Here's how the part is built. I have some questions about the finished solid (model axes, mm). A direction names the side the tool comes from. Coordinates: 2 decimals unless noted, no trailing zeros. Write each loop counter-clockwise with the first axis right and the second up, starting at its lowest first coordinate (ties: lowest second). Pieces come first, ordered by that corner, then holes.
```python
from build123d import *

# Parameters (mm, degrees)
BOSS_EXTRUDE1_DEPTH = 8
CIRPATTERN1_COUNT   = 4


# Read off the part's stored shape, not the designer's step: CSK for M3 Hex Socket Countersunk Cap Screw1
with BuildPart() as part:
    # Sketch2 → Boss-Extrude1 (new body)
    with BuildSketch(Plane(origin=(0, 0, 0), x_dir=(1, 0, 0), z_dir=(0, 1, 0))):
        with BuildLine():
            Line((6, -29.393876913), (102, -9.797958971))
            ThreePointArc((102, -9.797958971), (110, 0), (102, 9.797958971))
            Line((102, 9.797958971), (6, 29.393876913))
            ThreePointArc((6, 29.393876913), (-30, 0), (6, -29.393876913))
        make_face()
        with BuildLine():
            Line((37.941125497, -12.667714712), (100, 0))
            Line((100, 0), (37.941125497, 12.667714712))
            ThreePointArc((37.941125497, 12.667714712), (40, 0), (37.941125497, -12.667714712))
        make_face(mode=Mode.SUBTRACT)
    boss_extrude1 = extrude(amount=BOSS_EXTRUDE1_DEPTH)

    # CirPattern1: Boss-Extrude1 ×4 about axis
    cirpattern1_axis = Axis((0, 0, 0), (0, 1, 0))
    for i in range(1, CIRPATTERN1_COUNT):
        add(boss_extrude1.rotate(cirpattern1_axis, i * 360 / CIRPATTERN1_COUNT))

    # CSK for M3 Hex Socket Countersunk Ca 2 → CSK for M3 Hex Socket Countersunk Cap Screw1 (revolve, cut)
    with BuildSketch(Plane(origin=(-11.258330249, 0, -6.5), x_dir=(1, 0, 0), z_dir=(0, 0, 1))):
        Polygon((1.8, 1.56), (1.8, 8), (0, 8), (0, 0), (3.36, 0), align=None)
    revolve(axis=Axis((-11.258330249, 0, -6.5), (0, 1, 0)), mode=Mode.SUBTRACT)

    # CSK for M3 Hex Socket Countersunk Ca 3 o → CSK for M3 Hex Socket Countersunk Ca 3 (revolve, cut)
    with BuildSketch(Plane(origin=(-11.258330249, 0, 6.5), x_dir=(1, 0, 0), z_dir=(0, 0, 1))):
        Polygon((1.8, 1.56), (1.8, 8), (0, 8), (0, 0), (3.36, 0), align=None)
    revolve(axis=Axis((-11.258330249, 0, 6.5), (0, 1, 0)), mode=Mode.SUBTRACT)

    # CSK for M3 Hex Socket Countersunk Ca 4 o → CSK for M3 Hex Socket Countersunk Ca 4 (revolve, cut)
    with BuildSketch(Plane.XY.offset(13)):
        Polygon((1.8, 1.56), (1.8, 8), (0, 8), (0, 0), (3.36, 0), align=None)
    revolve(axis=Axis((0, 0, 13), (0, 1, 0)), mode=Mode.SUBTRACT)

    # CSK for M3 Hex Socket Countersunk Ca 5 o → CSK for M3 Hex Socket Countersunk Ca 5 (revolve, cut)
    with BuildSketch(Plane(origin=(11.258330249, 0, 6.5), x_dir=(1, 0, 0), z_dir=(0, 0, 1))):
        Polygon((1.8, 1.56), (1.8, 8), (0, 8), (0, 0), (3.36, 0), align=None)
    revolve(axis=Axis((11.258330249, 0, 6.5), (0, 1, 0)), mode=Mode.SUBTRACT)

    # CSK for M3 Hex Socket Countersunk Ca 6 o → CSK for M3 Hex Socket Countersunk Ca 6 (revolve, cut)
    with BuildSketch(Plane(origin=(11.258330249, 0, -6.5), x_dir=(1, 0, 0), z_dir=(0, 0, 1))):
        Polygon((1.8, 1.56), (1.8, 8), (0, 8), (0, 0), (3.36, 0), align=None)
    revolve(axis=Axis((11.258330249, 0, -6.5), (0, 1, 0)), mode=Mode.SUBTRACT)

    # CSK for M3 Hex Socket Countersunk Ca 7 o → CSK for M3 Hex Socket Countersunk Ca 7 (revolve, cut)
    with BuildSketch(Plane.XY.offset(-13)):
        Polygon((1.8, 1.56), (1.8, 8), (0, 8), (0, 0), (3.36, 0), align=None)
    revolve(axis=Axis((0, 0, -13), (0, 1, 0)), mode=Mode.SUBTRACT)


solid = part.part
```
1) Imagine slicing it at D-D on z = 29. Please give me the cut outline in (x, y), then the cut area to 3 significant figures.
Values follow:
outline: (-24.7, 0) - (24.7, 0) - (24.7, 8) - (-24.7, 8) - close
area: 395 mm2
2) Will these pins go through, and if not, where does the flat tip stop? pin 1 (4 mm diameter, centred on y = 2.5, z = -60, fed in from -X); pin 2 (1 mm diameter, centred on x = -7, y = 5, fed in from +Z); pin 3 (6 mm diameter, centred on x = -11.26, z = -6.5, fed in from +Y).
Values follow:
pin 1: stops at x = -18.78
pin 2: stops at z = 107.6
pin 3: stops at y = 8
3) On a 3-axis mill with a long thin cutter (end or side, diameter ignored), from which of +Z, -Z, +X, -X, +Y, -Y can I reach the whole of each face in a straight line? I mean faces 5 (the face through (69.405, 3.944, -6.245)), 6 (the face through (17.722, 3.944, -63.178)). Say none if no direction works.
Values follow:
face 5: +Y, -Y
face 6: -Z, +X, +Y, -Y
4) Imagine slicing it at A-A on x = 96. Please give me the cut outline in (y, z).
Values follow:
outline: (0, -11.02) - (8, -11.02) - (8, -0.82) - (0, -0.82) - close; (0, 0.82) - (8, 0.82) - (8, 11.02) - (0, 11.02) - close
5) We'd pull the mould along X, two halves only. Please class faces 1 (the face through (-68.54, 3.94, -6.42)), 2 (the face through (-17.504, 3.944, -64.25)), 3 (the face through (0, 4, -110)), 4 (the face through (68.54, 3.94, 6.42)): pulls with the +X half, pulls with the -X half, needs draft (parallel to the pull), parting line crosses it, or undercut.
Values follow:
face 1: undercut
face 2: pulls with the -X half
face 3: parting line crosses it
face 4: undercut
6) Imagine slicing it at B-B on y = 5. Count the separate pieces of the cut face and the enclosed holes in it, then the cut area to 3 significant figures.
Values follow:
separate pieces: 1
enclosed holes: 10
area: 10,800 mm2
7) I need wall thicknesses on probe 1 along Z at (x, y) = (-57, 0.5); probe 2 along X at (y, z) = (1.25, -78); probe 3 along X at (y, z) = (6.5, 68). Which ranges of each line are inside material? Lowest first, please.
Values follow:
probe 1: z = -18.98 to -8.78, 8.78 to 18.98
probe 2: x = -14.7 to -4.49, 4.49 to 14.7
probe 3: x = -16.74 to -6.53, 6.53 to 16.74
8) Imagine slicing it at C-C on z = -51.5. Please give me the cut outline in (x, y).
Values follow:
outline: (-20.11, 0) - (-9.9, 0) - (-9.9, 8) - (-20.11, 8) - close; (9.9, 0) - (20.11, 0) - (20.11, 8) - (9.9, 8) - close
